CAD build for the part. Positions are in the model's coordinates, mm. A direction names the side the tool comes from. Give positions to 0.01 mm unless a question says otherwise; leave off trailing zeros. Write each loop counter-clockwise with the first axis right and the second up, starting at its lowest first coordinate (ties: lowest second). Pieces come first, ordered by that corner, then holes. Notation, with made-up numbers: (58, 41) -> (104, 41) arc R33 cw to (104, 73) -> close; hole circle Ø5 at (63, 51). An arc over 180 degrees is marked (long way). Answer as a JSON object with one key per item and string values.
```python
from build123d import *

# Parameters (mm, degrees)
SKETCH1_W           = 19.05
SKETCH1_H           = 19.05
BOSS_EXTRUDE1_DEPTH = 9.525
FILLET1_R           = 1.27
SKETCH2_W           = 24.13
SKETCH2_H           = 24.13
BOSS_EXTRUDE2_DEPTH = 1.27
FILLET2_R           = 0.508
SKETCH3_W           = 16.51
SKETCH3_H           = 16.51
CUT_EXTRUDE2_DEPTH  = 8.89
SKETCH4_R           = 0.3175
CUT_EXTRUDE3_DEPTH  = 33.830175525


with BuildPart() as part:
    # Sketch1 → Boss-Extrude1 (new body)
    with BuildSketch(Plane(origin=(0, 0, 0), x_dir=(1, 0, 0), z_dir=(0, 1, 0))):
        with Locations((9.525, 9.525)):
            Rectangle(SKETCH1_W, SKETCH1_H)
    extrude(amount=BOSS_EXTRUDE1_DEPTH)

    # Fillet1
    fillet1_edges = [part.edges().sort_by_distance(p)[0] for p in [
        (19.05, 9.525, -9.525),
        (9.525, 9.525, -19.05),
        (0, 9.525, -9.525),
        (9.525, 9.525, 0),
    ]]
    fillet(fillet1_edges, radius=FILLET1_R)

    # Sketch2 → Boss-Extrude2 (add)
    with BuildSketch(Plane.XZ):
        with Locations((9.525, -9.525)):
            Rectangle(SKETCH2_W, SKETCH2_H)
    extrude(amount=BOSS_EXTRUDE2_DEPTH)

    # Fillet2
    fillet2_edges = [part.edges().sort_by_distance(p)[0] for p in [
        (21.59, 0, -9.525),
        (9.525, 0, 2.54),
        (-2.54, 0, -9.525),
        (9.525, 0, -21.59),
        (9.525, 0, -19.05),
        (19.05, 0, -9.525),
        (9.525, 0, 0),
        (0, 0, -9.525),
    ]]
    fillet(fillet2_edges, radius=FILLET2_R)

    # Sketch3 → Cut-Extrude2 (cut)
    with BuildSketch(Plane.XZ.offset(1.27)):
        with Locations((9.525, -9.525)):
            Rectangle(SKETCH3_W, SKETCH3_H)
    extrude(amount=-CUT_EXTRUDE2_DEPTH, mode=Mode.SUBTRACT)

    # Mirror3: part across plane


with BuildPart() as part_1:
    add(part.part)
    add(part.part.mirror(Plane(origin=(0, -1.27, 0), x_dir=(0, 0, 1), z_dir=(0, -1, 0))))

    # Sketch4 → Cut-Extrude3 (cut, through all)
    with BuildSketch(Plane(origin=(0, 0, 0), x_dir=(1, 0, 0), z_dir=(0, 1, 0))):
        with Locations(Location((20.32, 9.525, 0), (0, 0, 270))):
            Circle(SKETCH4_R)
        with Locations(Location((-1.27, 9.525, 0), (0, 0, 270))):
            Circle(SKETCH4_R)
    extrude(amount=-CUT_EXTRUDE3_DEPTH, mode=Mode.SUBTRACT)


solid = part_1.part
```
1) Slice it at C-C (y = 4.5). List the corners of the cut face in (x, z).
Model answer:
{"outline": "(0, -19.05) -> (19.05, -19.05) -> (19.05, 0) -> (0, 0) -> close; hole (1.27, -17.78) -> (17.78, -17.78) -> (17.78, -1.27) -> (1.27, -1.27) -> close"}
2) Slice it at B-B (x = 14). List the corners of the cut face in (y, z) (3 decimals), then the cut area to 3 significant figures.
Model answer:
{"outline": "(-12.065, -17.78) arc R1.27 ccw to (-10.795, -19.05) -> (-3.048, -19.05) arc R0.508 cw to (-2.54, -19.558) -> (-2.54, -21.082) arc R0.508 ccw to (-2.032, -21.59) -> (-0.508, -21.59) arc R0.508 ccw to (0, -21.082) -> (0, -19.558) arc R0.508 cw to (0.508, -19.05) -> (8.255, -19.05) arc R1.27 ccw to (9.525, -17.78) -> (9.525, -1.27) arc R1.27 ccw to (8.255, 0) -> (0.508, 0) arc R0.508 cw to (0, 0.508) -> (0, 2.032) arc R0.508 ccw to (-0.508, 2.54) -> (-2.032, 2.54) arc R0.508 ccw to (-2.54, 2.032) -> (-2.54, 0.508) arc R0.508 cw to (-3.048, 0) -> (-10.795, 0) arc R1.27 ccw to (-12.065, -1.27) -> close; hole (-10.16, -17.78) -> (7.62, -17.78) -> (7.62, -1.27) -> (-10.16, -1.27) -> close", "area": "129 mm2"}
3) Mould opens along Y. For faces 5 (the flat face through (9, -1, -1.27)), 6 (the flat face through (9, 9.525, -10)), 7 (the flat face through (0, -7, -9)) say: released by +Y, released by -Y, zero draft, split by the parting line, or undercut.
Model answer:
{"face 5": "undercut", "face 6": "released by +Y", "face 7": "zero draft"}
4) Slice it at D-D (z = -12.75). List the corners of the cut face in (x, y) (3 decimals).
Model answer:
{"outline": "(-2.54, -2.032) arc R0.508 ccw to (-2.032, -2.54) -> (-0.508, -2.54) arc R0.508 cw to (0, -3.048) -> (0, -10.795) arc R1.27 ccw to (1.27, -12.065) -> (17.78, -12.065) arc R1.27 ccw to (19.05, -10.795) -> (19.05, -3.048) arc R0.508 cw to (19.558, -2.54) -> (21.082, -2.54) arc R0.508 ccw to (21.59, -2.032) -> (21.59, -0.508) arc R0.508 ccw to (21.082, 0) -> (19.558, 0) arc R0.508 cw to (19.05, 0.508) -> (19.05, 8.255) arc R1.27 ccw to (17.78, 9.525) -> (1.27, 9.525) arc R1.27 ccw to (0, 8.255) -> (0, 0.508) arc R0.508 cw to (-0.508, 0) -> (-2.032, 0) arc R0.508 ccw to (-2.54, -0.508) -> close; hole (1.27, -10.16) -> (17.78, -10.16) -> (17.78, 7.62) -> (1.27, 7.62) -> close"}
5) 3-axis set-ups, long thin cutter, end or side, ignore diameter. For faces 1 (the flat face through (9, -7, 0)), 2 (the flat face through (9, 4, -19.05)), 3 (the flat face through (19.05, 4, -9)), 4 (the flat face through (9, 7.62, -9)): which of +Z, -Z, +X, -X, +Y, -Y reach the whole face in a straight line?
Model answer:
{"face 1": "+Z, +X, -X, -Y", "face 2": "-Z, +X, -X, +Y", "face 3": "+Z, -Z, +X, +Y", "face 4": "none"}
6) Pin check, flat tips, straight feed: pin 1 (5 mm diameter, centred on x = 1, y = 3.5, fed in from +Z); pin 2 (3 mm diameter, centred on y = 5.5, z = -10.5, fed in from -X); pin 3 (2.5 mm diameter, centred on y = 5.5, z = -12.5, fed in from +X). Stop position of each tip, or through.
Model answer:
{"pin 1": "stops at z = 0", "pin 2": "stops at x = 0", "pin 3": "stops at x = 19.05"}
7) Slice it at A-A (y = -1). List the corners of the cut face in (x, z) (1 decimal).
Model answer:
{"outline": "(-2.5, -21.6) -> (21.6, -21.6) -> (21.6, 2.5) -> (-2.5, 2.5) -> close; hole circle Ø0.6 at (-1.3, -9.5); hole (1.3, -17.8) -> (17.8, -17.8) -> (17.8, -1.3) -> (1.3, -1.3) -> close; hole circle Ø0.6 at (20.3, -9.5)"}
8) Wall check: probe 1 along Z at (x, y) = (6.5, -2); probe 2 along X at (y, z) = (5, -15); probe 3 along Z at (x, y) = (17, 5.25). Give the ranges that are in metal, low to high.
Model answer:
{"probe 1": "z = -21.59 to -17.78, -1.27 to 2.54", "probe 2": "x = 0 to 1.27, 17.78 to 19.05", "probe 3": "z = -19.05 to -17.78, -1.27 to 0"}
